Geometry: final body of the model. Coordinates: model frame, mm. Face numbers are marked on the shaded views. Round coordinates to 2 decimals unless told otherwise and drop trailing zeros. Write each loop counter-clockwise with the first axis right and the second up, starting at its lowest first coordinate (ties: lowest second). Pieces come first, ordered by that corner, then holes. Notation, with made-up numbers: M -34,16.25 L -15,16.25 A16 cw -15,28.25 Z; hole C 39,61.5 d11. An arc over 180 degrees is marked long. Put each result on its own line as item: value. Start each with the question number.
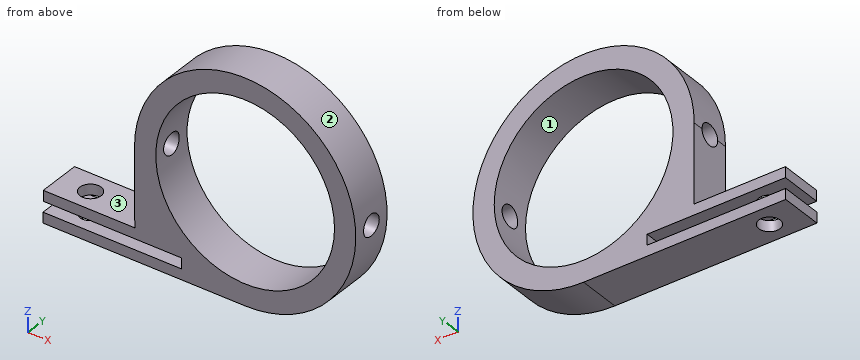
```python
from build123d import *

# Parameters (mm, degrees)
PAD_DEPTH            = 20
SKETCH002_R          = 5
POCKET001_DEPTH      = 104.001
HOLE001_D            = 6.6
HOLE001_DEPTH        = 25
HOLE001_CSINK_D      = 12
HOLE001_CSINK_ANGLE  = 90
HOLE001_TIPS_R       = 3.3
SKETCH001_R          = 42
POCKET_DEPTH         = 20.001
SKETCH020_R          = 5
POCKET005_DEPTH      = 15.001
BODY_PLACEMENT_ANGLE = 90


with BuildPart() as part:
    # Sketch → Pad (new body)
    with BuildSketch(Plane.XY):
        with BuildLine():
            Line((-51.87, -37), (-94.87, -37))
            Line((-94.87, -37), (-94.87, -42))
            Line((-94.87, -42), (-29.87, -42))
            Line((-29.87, -42), (-29.87, -47))
            Line((-29.87, -47), (-95, -47))
            Line((-95, -47), (-95, -52))
            Line((-95, -52), (-30, -52))
            Line((-30, -52), (0, -52))
            ThreePointArc((0, -52), (36.769553, 36.769553), (-52, 0))
            Line((-52, 0), (-51.87, -37))
        make_face()
    extrude(amount=PAD_DEPTH)

    # Sketch002 (on DatumPlane) → Pocket001 (cut, through all)
    with BuildSketch(Plane(origin=(-52, 0, 0), x_dir=(0, -1, 0), z_dir=(-1, 0, 0))):
        with Locations((0, 10)):
            Circle(SKETCH002_R)
    extrude(amount=-POCKET001_DEPTH, mode=Mode.SUBTRACT)

    # Hole001
    with Locations(Plane.XZ.offset(42)):
        with Locations((65, 10)):
            CounterSinkHole(HOLE001_D / 2, HOLE001_CSINK_D / 2, depth=HOLE001_DEPTH, counter_sink_angle=HOLE001_CSINK_ANGLE)

    # Hole001 tips → Hole001 tip 1 section 0
    with BuildSketch(Plane.XZ.offset(17), mode=Mode.PRIVATE) as hole001_tip_1_s0:
        with Locations((65, 10)):
            Circle(HOLE001_TIPS_R)
    loft([hole001_tip_1_s0.sketch, Vertex(65, -15.01716, 10)], mode=Mode.SUBTRACT)

    # Sketch001 → Pocket (cut, through all)
    with BuildSketch(Plane.XY.offset(20)):
        Circle(SKETCH001_R)
    extrude(amount=-POCKET_DEPTH, mode=Mode.SUBTRACT)

    # Sketch020 (on DatumPlane) → Pocket005 (cut, through all)
    with BuildSketch(Plane(origin=(0, -37, 0), x_dir=(-1, 0, 0), z_dir=(0, 1, 0))):
        with Locations((80, 10)):
            Circle(SKETCH020_R)
    extrude(amount=-POCKET005_DEPTH, mode=Mode.SUBTRACT)


with BuildPart() as part_1:
    # Body placement: moved
    add(part.part.moved(Location((1, -773, 0))).rotate(Axis((1, -773, 0), (1, 0, 0)), BODY_PLACEMENT_ANGLE))


solid = part_1.part
```
1) Section C-C, the plane y = -775.5. Output: boundary loops of the cut face in (x, z), and give its area (3 significant figures).
2) First-contact query: pin 1 (3 mm diameter, centred on y = -788, z = 0.5, fed in from -X); pin 2 (10 mm diameter, centred on x = -69.5, y = -786.5, fed in from +Z); pin 3 (1.5 mm diameter, centred on y = -788, z = -40, fed in from -X); pin 4 (6 mm diameter, centred on y = -783, z = 0, fed in from +X). Flat tips, straight axial feed; report the tip coordinate or a pass-through.
3) Draft query along X for the marked faces 1, 2 and 3. Return one class per face: +X half, -X half, draft (parallel to the pull), parting line (faces both ways), or undercut.
4) Section B-B, the plane x = -44. Output: boundary loops of the cut face in (y, z), and give its area (3 significant figures).
5) Ray query, probe 1 along Y at (x, z) = (-79, -39.5); probe 2 along Z at (x, y) = (-55.5, -775); probe 3 along Z at (x, y) = (-35, -790.75). Return the intervals inside material, ascending.
6) Section D-D, the plane y = -783. Output: boundary loops of the cut face in (x, z).
7) Section A-A, the plane x = -79. Output: boundary loops of the cut face in (y, z).
Solved:
1. outline: M -94,-52 L 1,-52 A52 ccw long -51,0 L -50.87,-37 L -93.87,-37 L -93.87,-42 L -28.87,-42 L -28.87,-47 L -94,-47 Z; hole C 1,0 d84
1. area: 3,850 mm2
2. pin 1: stops at x = -51
2. pin 2: stops at z = -37
2. pin 3: stops at x = -93.87
2. pin 4: passes through
3. face 1: undercut
3. face 2: parting line
3. face 3: draft
4. outline: M -793,-52 L -773,-52 L -773,-47 L -793,-47 Z; M -793,-42 L -773,-42 L -773,26.06 L -793,26.06 Z; hole C -783,0 d10
4. area: 1,380 mm2
5. probe 1: y = -793 to -788, -778 to -773
5. probe 2: z = -52 to -47, -42 to -37
5. probe 3: z = -52 to -47, -42 to -21.63, 21.63 to 37.52
6. outline: M -94,-52 L -84,-52 L -84,-47 L -94,-47 Z; M -93.87,-42 L -84,-42 L -84,-37 L -93.87,-37 Z; M -74,-52 L 1,-52 A52 ccw 52.76,-5 L 42.7,-5 A42 cw -40.7,-5 L -50.98,-5 L -50.87,-37 L -74,-37 L -74,-42 L -28.87,-42 L -28.87,-47 L -74,-47 Z; M -50.76,5 L -40.7,5 A42 cw 42.7,5 L 52.76,5 A52 ccw Z
7. outline: M -793,-52 L -788,-52 L -788,-47 L -793,-47 Z; M -793,-42 L -788,-42 L -788,-37 L -793,-37 Z; M -778,-52 L -773,-52 L -773,-47 L -778,-47 Z; M -778,-42 L -773,-42 L -773,-37 L -778,-37 Z
